from build123d import *

# Parameters (mm, degrees)
F0_W     = 76.2
F0_H     = 38.1
F1_DEPTH = 25.4
F2_R     = 11.1125
F3_DEPTH = 12.7
F4_T     = -7.9375
F5_R     = 3.175
F6_DEPTH = 38.1
F7_SIZE2 = 3.175
F7_SIZE  = 3.175


with BuildPart() as f1:
    # F0 (on Top) → F1 (new body)
    with BuildSketch(Plane.XY):
        with Locations((38.1, 19.05)):
            Rectangle(F0_W, F0_H)
    extrude(amount=F1_DEPTH)

    # F2 (on face) → F3 (join)
    with BuildSketch(Plane.XY.offset(25.4)):
        with Locations((19.05, 19.05)):
            Circle(F2_R)
        with Locations((57.15, 19.05)):
            Circle(F2_R)
    extrude(amount=F3_DEPTH)

    # F4
    f4_openings = [f1.faces().sort_by_distance(p)[0] for p in [
        (38.1, 19.05, 0),
    ]]
    offset(amount=F4_T, openings=f4_openings, kind=Kind.INTERSECTION)

    # F5 (on face) → F6 (cut)
    with BuildSketch(Plane.XZ):
        with Locations((38.1, 12.7)):
            Circle(F5_R)
    extrude(amount=-F6_DEPTH, mode=Mode.SUBTRACT)

    # F7
    f7_edges = [f1.edges().sort_by_distance(p)[0] for p in [
        (7.9375, 19.05, 38.1),
        (46.0375, 19.05, 38.1),
        (38.1, 0, 25.4),
        (0, 19.05, 25.4),
        (38.1, 38.1, 25.4),
        (76.2, 19.05, 25.4),
    ]]
    chamfer(f7_edges, length=F7_SIZE, length2=F7_SIZE2)


solid = f1.part
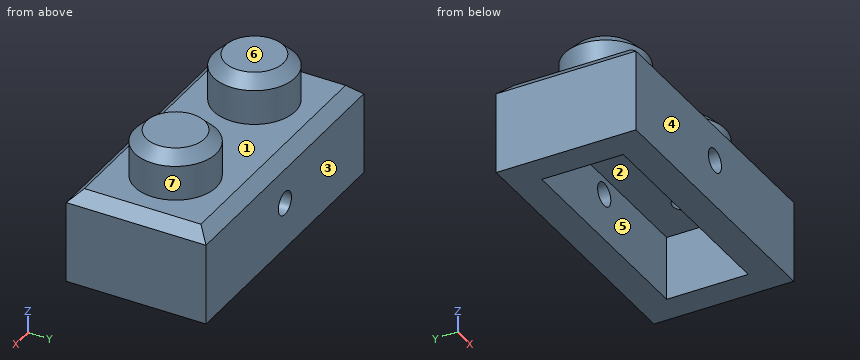
The listing builds one solid part. Answer for the finished solid, in the listing's coordinates (mm). Face numbers are marked on the shaded views. A direction names the side the tool comes from. Give positions to 0.01 mm unless a question says otherwise; leave off trailing zeros. Loops run counter-clockwise (first coordinate to the right, second up) from the corner with the lowest first, then second, coordinate; pieces in that order, holes last. Notation, with made-up numbers: (79.25, -4) - (130.25, -4) arc R21 cw to (130.25, 28) - close; hole circle Ø8 at (-30.5, -20). An arc over 180 degrees is marked (long way). Write each question's results on one line, items separated by ' | '.
1. Find section D-D, the plane z = 12.7. Write down the section's boundary in (x, y) (1 decimal).
Resolved:
outline: (0, 0) - (34.9, 0) - (34.9, 7.9) - (7.9, 7.9) - (7.9, 30.2) - (34.9, 30.2) - (34.9, 38.1) - (0, 38.1) - close; (41.3, 0) - (76.2, 0) - (76.2, 38.1) - (41.3, 38.1) - (41.3, 30.2) - (68.3, 30.2) - (68.3, 7.9) - (41.3, 7.9) - close
2. Consider probe 1 along Y at (x, z) = (14, 9.5); probe 2 along X at (y, z) = (27, 14); probe 3 along X at (y, z) = (18, 25.5). Determine where each line is inside the solid, lowest interval first. Write a range as from..to.
Resolved:
probe 1: y = 0..7.94, 30.16..38.1 | probe 2: x = 0..7.94, 68.26..76.2 | probe 3: x = 7.99..16.05, 22.05..30.11, 46.09..54.15, 60.15..68.21
3. Find section C-C, the plane y = 5.5. Write down the section's boundary in (x, z) (3 decimals).
Resolved:
outline: (0, 0) - (76.2, 0) - (76.2, 22.225) - (73.025, 25.4) - (3.175, 25.4) - (0, 22.225) - close; hole circle Ø6.35 at (38.1, 12.7)
4. Which of the six approach directions +Z, -Z, +X, -X, +Y, -Y give full straight-line access (tool end or side, diameter ignored) to the marked faces 1, 2 and 3?
Resolved:
face 1: +Z | face 2: -Z | face 3: +Z, -Z, +X, -X, +Y
5. Flat-ended cylindrical pins translate along their axes: P1, Ø3, axis at x = 18, y = 18, coming from the -Z side; P2, Ø12, axis at x = 48.5, z = 28.5, coming from the +Y side (3 decimals); P3, Ø4, axis at x = 18.5, y = 27, coming from the -Z side. Find the tip coordinate at first contact, or state that the pin passes through.
Resolved:
P1: stops at z = 30.16 | P2: stops at y = 37.825 | P3: stops at z = 17.46
6. Find section A-A, the plane z = 2. Write down the section's boundary in (x, y), then the cut area to 3 significant figures.
Resolved:
outline: (0, 0) - (76.2, 0) - (76.2, 38.1) - (0, 38.1) - close; hole (7.94, 7.94) - (68.26, 7.94) - (68.26, 30.16) - (7.94, 30.16) - close | area: 1,560 mm^2
7. For a pull along Y with two mould halves and no side action, classify the marked faces 4, 5, 6 and 7 as +Y half, -Y half, draft (parallel to the pull), parting line (faces both ways), or undercut.
Resolved:
face 4: -Y half | face 5: undercut | face 6: draft | face 7: parting line
8. Find section B-B, the plane x = 33. Write down the section's boundary in (y, z) (1 decimal).
Resolved:
outline: (0, 0) - (7.9, 0) - (7.9, 17.5) - (30.2, 17.5) - (30.2, 0) - (38.1, 0) - (38.1, 22.2) - (34.9, 25.4) - (3.2, 25.4) - (0, 22.2) - close
